The model under review builds one solid part; all positions refer to its coordinate system, in mm. Coordinates: 2 decimals unless noted, no trailing zeros. Order: outer loops, then holes, each group sorted by start corner. A loop starts at its lowest first (then second) coordinate and runs counter-clockwise, first axis right, second up. Notation, with made-up numbers: (36, 74) - (52, 74) arc R32 cw to (52, 107) - close; hole circle Ø11 at (17.5, 13.25). An arc over 180 degrees is marked (long way). Answer in a Markdown table with one row per item.
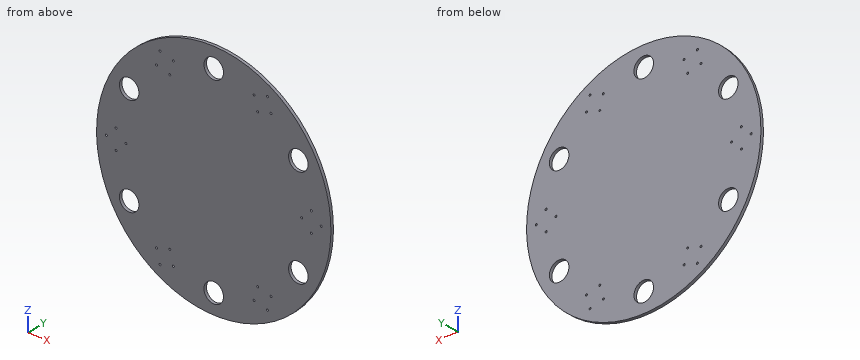
```python
from build123d import *

# Parameters (mm, degrees)
SKETCH1_R           = 120
SKETCH1_R_2         = 1
SKETCH1_R_3         = 10
BOSS_EXTRUDE1_DEPTH = 3


with BuildPart() as part:
    # Sketch1 → Boss-Extrude1 (new body)
    with BuildSketch(Plane(origin=(0, 0, 0), x_dir=(1, 0, 0), z_dir=(0, 1, 0))):
        with Locations(Location((0, 0, 0), (0, 0, 270))):
            Circle(SKETCH1_R)
        with Locations(Location((45, -77.942286341, 0), (0, 0, 270))):
            Circle(SKETCH1_R_2, mode=Mode.SUBTRACT)
        with Locations(Location((58.660254038, -81.602540378, 0), (0, 0, 270))):
            Circle(SKETCH1_R_2, mode=Mode.SUBTRACT)
        with Locations(Location((55, -95.262794416, 0), (0, 0, 270))):
            Circle(SKETCH1_R_2, mode=Mode.SUBTRACT)
        with Locations(Location((41.339745962, -91.602540378, 0), (0, 0, 270))):
            Circle(SKETCH1_R_2, mode=Mode.SUBTRACT)
        with Locations(Location((110, 0, 0), (0, 0, 270))):
            Circle(SKETCH1_R_2, mode=Mode.SUBTRACT)
        with Locations(Location((100, -10, 0), (0, 0, 270))):
            Circle(SKETCH1_R_2, mode=Mode.SUBTRACT)
        with Locations(Location((90, 0, 0), (0, 0, 270))):
            Circle(SKETCH1_R_2, mode=Mode.SUBTRACT)
        with Locations(Location((100, 10, 0), (0, 0, 270))):
            Circle(SKETCH1_R_2, mode=Mode.SUBTRACT)
        with Locations(Location((-45, -77.942286341, 0), (0, 0, 270))):
            Circle(SKETCH1_R_2, mode=Mode.SUBTRACT)
        with Locations(Location((-41.339745962, -91.602540378, 0), (0, 0, 270))):
            Circle(SKETCH1_R_2, mode=Mode.SUBTRACT)
        with Locations(Location((-55, -95.262794416, 0), (0, 0, 270))):
            Circle(SKETCH1_R_2, mode=Mode.SUBTRACT)
        with Locations(Location((-58.660254038, -81.602540378, 0), (0, 0, 270))):
            Circle(SKETCH1_R_2, mode=Mode.SUBTRACT)
        with Locations(Location((-90, 0, 0), (0, 0, 270))):
            Circle(SKETCH1_R_2, mode=Mode.SUBTRACT)
        with Locations(Location((-100, -10, 0), (0, 0, 270))):
            Circle(SKETCH1_R_2, mode=Mode.SUBTRACT)
        with Locations(Location((-110, 0, 0), (0, 0, 270))):
            Circle(SKETCH1_R_2, mode=Mode.SUBTRACT)
        with Locations(Location((-100, 10, 0), (0, 0, 270))):
            Circle(SKETCH1_R_2, mode=Mode.SUBTRACT)
        with Locations(Location((-45, 77.942286341, 0), (0, 0, 270))):
            Circle(SKETCH1_R_2, mode=Mode.SUBTRACT)
        with Locations(Location((-58.660254038, 81.602540378, 0), (0, 0, 270))):
            Circle(SKETCH1_R_2, mode=Mode.SUBTRACT)
        with Locations(Location((-55, 95.262794416, 0), (0, 0, 270))):
            Circle(SKETCH1_R_2, mode=Mode.SUBTRACT)
        with Locations(Location((-41.339745962, 91.602540378, 0), (0, 0, 270))):
            Circle(SKETCH1_R_2, mode=Mode.SUBTRACT)
        with Locations(Location((45, 77.942286341, 0), (0, 0, 270))):
            Circle(SKETCH1_R_2, mode=Mode.SUBTRACT)
        with Locations(Location((41.339745962, 91.602540378, 0), (0, 0, 270))):
            Circle(SKETCH1_R_2, mode=Mode.SUBTRACT)
        with Locations(Location((55, 95.262794416, 0), (0, 0, 270))):
            Circle(SKETCH1_R_2, mode=Mode.SUBTRACT)
        with Locations(Location((58.660254038, 81.602540378, 0), (0, 0, 270))):
            Circle(SKETCH1_R_2, mode=Mode.SUBTRACT)
        with Locations(Location((0, 100, 0), (0, 0, 270))):
            Circle(SKETCH1_R_3, mode=Mode.SUBTRACT)
        with Locations(Location((-86.602540378, 50, 0), (0, 0, 270))):
            Circle(SKETCH1_R_3, mode=Mode.SUBTRACT)
        with Locations(Location((-86.602540378, -50, 0), (0, 0, 270))):
            Circle(SKETCH1_R_3, mode=Mode.SUBTRACT)
        with Locations(Location((0, -100, 0), (0, 0, 270))):
            Circle(SKETCH1_R_3, mode=Mode.SUBTRACT)
        with Locations(Location((86.602540378, -50, 0), (0, 0, 270))):
            Circle(SKETCH1_R_3, mode=Mode.SUBTRACT)
        with Locations(Location((86.602540378, 50, 0), (0, 0, 270))):
            Circle(SKETCH1_R_3, mode=Mode.SUBTRACT)
    extrude(amount=BOSS_EXTRUDE1_DEPTH)


solid = part.part
```
Item 1: We need section A-A, the plane x = -83.5. Write out the cut boundary in (y, z).
Check values:
| item | result |
|---|---|
| outline | (0, -86.18) - (3, -86.18) - (3, -59.51) - (0, -59.51) - close; (0, -40.49) - (3, -40.49) - (3, 40.49) - (0, 40.49) - close; (0, 59.51) - (3, 59.51) - (3, 86.18) - (0, 86.18) - close |
Item 2: Clearance check with flat-ended pins moving along their axes: pin 1 Ø1.2 at (x, z) = (41.34, 91.6) entering from -Y; pin 2 Ø1.5 at (y, z) = (2, -78) entering from +X; pin 3 Ø1 at (y, z) = (1.5, 28) entering from -X. State where each tip first meets the part, or that it passes through.
Check values:
| item | result |
|---|---|
| pin 1 | through |
| pin 2 | x = 91.83 |
| pin 3 | x = -116.81 |
Item 3: To check wall thickness, follow line 1 (Z direction, x = -89.5, y = 2.4); line 2 (X direction, y = 1.8, z = -52); line 3 (Z direction, x = -90, y = 1.2). State the ranges of each line that lie inside material, in increasing order. Write a range as from..to.
Check values:
| item | result |
|---|---|
| line 1 | -79.94..-59.57, -40.43..-0.87, 0.87..40.43, 59.57..79.94 |
| line 2 | -108.15..-96.4, -76.8..76.8, 96.4..108.15 |
| line 3 | -79.37..-59.41, -40.59..-1, 1..40.59, 59.41..79.37 |
Item 4: We need section C-C, the plane z = 100. Write out the cut boundary in (x, y).
Check values:
| item | result |
|---|---|
| outline | (-66.33, 0) - (-10, 0) - (-10, 3) - (-66.33, 3) - close; (10, 0) - (66.33, 0) - (66.33, 3) - (10, 3) - close |
Item 5: We need section B-B, the plane y = 0.7. State how many separate pieces and enclosed holes the cut face has, then the cut area to 3 significant figures.
Check values:
| item | result |
|---|---|
| separate pieces | 1 |
| enclosed holes | 30 |
| area | 43,300 mm^2 |
Item 6: We need section D-D, the plane z = -63.5. Write out the cut boundary in (x, y), then the cut area to 3 significant figures.
Check values:
| item | result |
|---|---|
| outline | (-101.82, 0) - (101.82, 0) - (101.82, 3) - (-101.82, 3) - close |
| area | 611 mm^2 |
